Input: dimensioned drawing with shaded views. Units: mm. Origin: part minimum x, y, z. Round coordinates to 2 decimals unless told otherwise and drop trailing zeros. Loops run counter-clockwise (first coordinate to the right, second up) from the corner with the lowest first, then second, coordinate; pieces in that order, holes last.
1) Section B-B, the plane x = 1.5. Return loops of the section in (y, z), and give its area (3 significant figures).
2) Section C-C, the plane y = 1.05. Return loops of the section in (x, z), and give its area (3 significant figures).
3) Section D-D, the plane z = 18.75. Return loops of the section in (x, y).
4) Section A-A, the plane z = 33. Return loops of the section in (x, y), and give its area (3 significant figures).
5) Ray query, line 1 along Z through (x, y) = (34.5, 1.3); line 2 along X through (y, z) = (0.35, 31); line 3 along Z through (x, y) = (20, 1.9). Return the intervals inside material, ascending.
6) First-contact query: pin 1 (1.5 mm diameter, centred on y = 2, z = 30, fed in from +X); pin 2 (0.9 mm diameter, centred on x = 1, y = 2, fed in from -Z); pin 3 (1.5 mm diameter, centred on y = 1, z = 29, fed in from -X); pin 4 (8 mm diameter, centred on x = 13.5, z = 28, fed in from -Y). Flat tips, straight axial feed; report the tip coordinate or a pass-through.
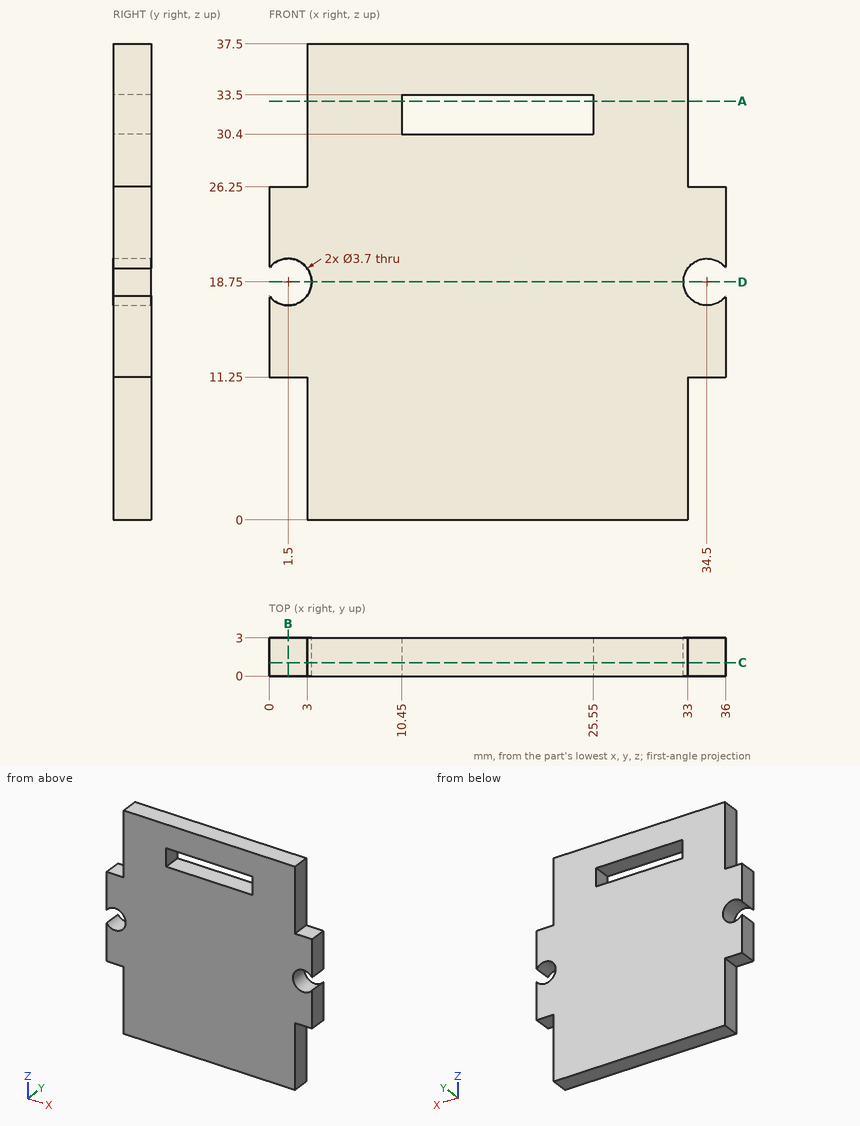
Final values:
1. outline: (0, 11.25) - (3, 11.25) - (3, 16.9) - (0, 16.9) - close; (0, 20.6) - (3, 20.6) - (3, 26.25) - (0, 26.25) - close
1. area: 33.9 mm2
2. outline: (0, 11.25) - (3, 11.25) - (3, 0) - (33, 0) - (33, 11.25) - (36, 11.25) - (36, 17.67) arc R1.85 cw (long way) to (36, 19.83) - (36, 26.25) - (33, 26.25) - (33, 37.5) - (3, 37.5) - (3, 26.25) - (0, 26.25) - (0, 19.83) arc R1.85 cw (long way) to (0, 17.67) - close; hole (10.45, 30.4) - (25.55, 30.4) - (25.55, 33.5) - (10.45, 33.5) - close
2. area: 1,150 mm2
3. outline: (3.35, 0) - (32.65, 0) - (32.65, 3) - (3.35, 3) - close
4. outline: (3, 0) - (10.45, 0) - (10.45, 3) - (3, 3) - close; (25.55, 0) - (33, 0) - (33, 3) - (25.55, 3) - close
4. area: 44.7 mm2
5. line 1: z = 11.25 to 16.9, 20.6 to 26.25
5. line 2: x = 3 to 10.45, 25.55 to 33
5. line 3: z = 0 to 30.4, 33.5 to 37.5
6. pin 1: stops at x = 33
6. pin 2: stops at z = 11.25
6. pin 3: stops at x = 3
6. pin 4: stops at y = 0
